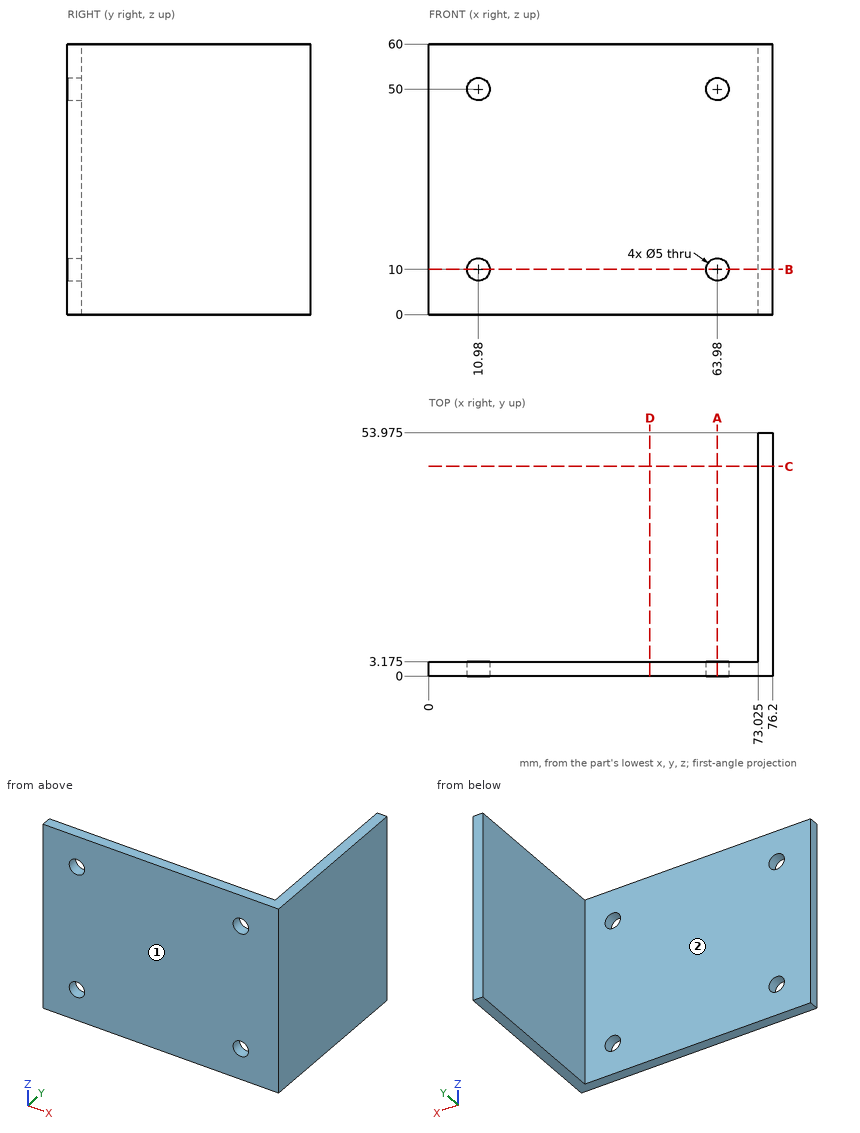
Design review of the part shown in the three views and the two pictorial views. Dimensions are in mm from the part's minimum x, y and z. A direction names the side the tool comes from. Round coordinates to 2 decimals unless told otherwise and drop trailing zeros. Write each loop counter-clockwise with the first axis right and the second up, starting at its lowest first coordinate (ties: lowest second). Pieces come first, ordered by that corner, then holes. Notation, with made-up numbers: (-18.5, 71.5) - (17.5, 71.5) arc R19 ccw to (17.5, 93.5) - close; hole circle Ø10 at (29, -5). An arc over 180 degrees is marked (long way). Return JSON: item names as keys, results as strings. Group by question number.
Item 1: For probe 1 along Z at (x, y) = (63.98, 1.7); probe 2 along X at (y, z) = (2.4, 50); probe 3 along Y at (x, z) = (28, 29) (3 decimals), list the stretches that pass through material, from the lowest coordinate up. Write a range as [from, to].
Item 2: We need section C-C on y = 46.5. Write out the cut boundary in (x, z) (3 decimals).
Item 3: Insertion check: P1, Ø1, axis at y = 31.5, z = 29, coming from the -X side (3 decimals); P2, Ø6.5, axis at x = 10.98, z = 10, coming from the +Y side (3 decimals); P3, Ø4.5, axis at x = 63.98, z = 10, coming from the -Y side; P4, Ø10, axis at x = 17.5, z = 53, coming from the -Y side. Each pin has a flat end and moves straight along its axis. Give the tip position at first contact, or say it passes through.
Item 4: We need section D-D on x = 49. Write out the cut boundary in (y, z) (3 decimals), and give its area (4 significant figures).
Item 5: Machinability: for the marked faces 1 and 2, which of the approach directions +Z, -Z, +X, -X, +Y, -Y give a long, thin tool a straight path to every point of the face, cutting with its end or side? Answer none if there is none.
Item 6: We need section B-B on z = 10. Write out the cut boundary in (x, y) (3 decimals), and give its area (3 significant figures).
Item 7: We need section A-A on x = 63.98. Write out the cut boundary in (y, z) (3 decimals).
Model answer:
{
 "1": {"probe 1": "z = [0, 7.5], [12.5, 47.5], [52.5, 60]", "probe 2": "x = [0, 8.48], [13.48, 61.48], [66.48, 76.2]", "probe 3": "y = [0, 3.175]"},
 "2": {"outline": "(73.025, 0) - (76.2, 0) - (76.2, 60) - (73.025, 60) - close"},
 "3": {"P1": "stops at x = 73.025", "P2": "stops at y = 3.175", "P3": "passes through", "P4": "stops at y = 0"},
 "4": {"outline": "(0, 0) - (3.175, 0) - (3.175, 60) - (0, 60) - close", "area": "190.5 mm²"},
 "5": {"face 1": "+Z, -Z, +X, -X, -Y", "face 2": "+Z, -Z, -X, +Y"},
 "6": {"outline": "(0, 0) - (8.48, 0) - (8.48, 3.175) - (0, 3.175) - close; (13.48, 0) - (61.48, 0) - (61.48, 3.175) - (13.48, 3.175) - close; (66.48, 0) - (76.2, 0) - (76.2, 53.975) - (73.025, 53.975) - (73.025, 3.175) - (66.48, 3.175) - close", "area": "371 mm²"},
 "7": {"outline": "(0, 0) - (3.175, 0) - (3.175, 7.5) - (0, 7.5) - close; (0, 12.5) - (3.175, 12.5) - (3.175, 47.5) - (0, 47.5) - close; (0, 52.5) - (3.175, 52.5) - (3.175, 60) - (0, 60) - close"}
}
